Part model, mm, in its own coordinate system. A direction names the side the tool comes from. Give positions to 0.01 mm unless a question says otherwise; leave off trailing zeros. Loops run counter-clockwise (first coordinate to the right, second up) from the corner with the lowest first, then second, coordinate; pieces in that order, holes last. Notation, with made-up numbers: M -20.5,-14.75 L 17.5,-14.75 A20 ccw 17.5,6.25 Z; hole C -14,63 d10. An arc over 180 degrees is marked long. Answer in a Markdown table with one row per item.
from build123d import *

# Parameters (mm, degrees)
CROQUIS1_R              = 3.175
SALIENTE_EXTRUIR1_DEPTH = 150
REDONDEO1_R             = 10
CORTAR_EXTRUIR1_DEPTH   = 13
REDONDEO2_R             = 5
CROQUIS3_W              = 98.791812306
CROQUIS3_H              = 18.145434914
CORTAR_EXTRUIR2_DEPTH   = 13.0000001
CORTAR_EXTRUIR3_DEPTH   = 3.0000001


with BuildPart() as part:
    # Croquis1 → Saliente-Extruir1 (new body)
    with BuildSketch(Plane.XY):
        with BuildLine():
            Line((-2, 19.285827964), (-8.98691391, 23.296314259))
            ThreePointArc((-8.98691391, 23.296314259), (-9.006535925, 33.69237342), (0, 28.5))
            Line((0, 28.5), (0, -28.5))
            ThreePointArc((0, -28.5), (-9.006535925, -33.69237342), (-8.98691391, -23.296314259))
            Line((-8.98691391, -23.296314259), (-2, -19.285827964))
            Line((-2, -19.285827964), (-2, 19.285827964))
        make_face()
        with Locations((-6, 28.5)):
            Circle(CROQUIS1_R, mode=Mode.SUBTRACT)
        with Locations((-6, -28.5)):
            Circle(CROQUIS1_R, mode=Mode.SUBTRACT)
    extrude(amount=-SALIENTE_EXTRUIR1_DEPTH)

    # Redondeo1
    redondeo1_edges = [part.edges().sort_by_distance(p)[0] for p in [
        (-2, -19.285827964, -75),
        (-2, 19.285827964, -75),
    ]]
    fillet(redondeo1_edges, radius=REDONDEO1_R)

    # Croquis2 → Cortar-Extruir1 (cut, through all)
    with BuildSketch(Plane(origin=(0, 0, 0), x_dir=(0, 0, -1), z_dir=(1, 0, 0))):
        Polygon((16, 25), (20, 15.646846929), (20, -15.646846929), (16, -25), (-29.873538988, -25), (-29.873538988, 25), align=None)
    extrude(amount=-CORTAR_EXTRUIR1_DEPTH, mode=Mode.SUBTRACT)

    # Redondeo2
    redondeo2_edges = [part.edges().sort_by_distance(p)[0] for p in [
        (-1.117074127, 15.646846929, -20),
        (-1.117074127, -15.646846929, -20),
        (-5.436698586, -25, -16),
        (-5.436698586, 25, -16),
    ]]
    fillet(redondeo2_edges, radius=REDONDEO2_R)

    # Croquis3 → Cortar-Extruir2 (cut, through all)
    with BuildSketch(Plane(origin=(0, 0, 0), x_dir=(0, 0, -1), z_dir=(1, 0, 0))):
        with Locations((75, 35.875128035)):
            Rectangle(CROQUIS3_W, CROQUIS3_H)
        with Locations((75, -35.875128035)):
            Rectangle(CROQUIS3_W, CROQUIS3_H)
    extrude(amount=-CORTAR_EXTRUIR2_DEPTH, mode=Mode.SUBTRACT)

    # Croquis4 → Cortar-Extruir3 (cut, through all)
    with BuildSketch(Plane.ZY.offset(2)):
        with BuildLine():
            Line((-143.359821197, 3), (-139.627206237, 3))
            ThreePointArc((-139.627206237, 3), (-136.627206237, 0), (-139.627206237, -3))
            Line((-139.627206237, -3), (-143.359821197, -3))
            ThreePointArc((-143.359821197, -3), (-146.359821197, 0), (-143.359821197, 3))
        make_face()
    extrude(amount=-CORTAR_EXTRUIR3_DEPTH, mode=Mode.SUBTRACT)


solid = part.part
(1) Drill centre lines: line 1 along Y through (x, z) = (-5.75, -136.5); line 2 along Z through (x, y) = (-2.5, 27.5); line 3 along Y through (x, z) = (-6, -95) (3 decimals). Where is each one in solid material? Low to high.
Recorded:
| item | result |
|---|---|
| line 1 | y = -34.49 to -31.67, -25.33 to -21.3, 21.3 to 25.33, 31.67 to 34.49 |
| line 2 | z = -150 to -124.4, -25.6 to 0 |
| line 3 | y = -25.325 to -21.496, 21.496 to 25.325 |
(2) Pull direction X, two halves, no side cores. Call faces 6 (the face through (-3.4, 18.6, -84.5)), 7 (the face through (-6.41, -25.35, -73.95)), 8 (the face through (-5, -25, -6)): +X half, -X half, draft (parallel to the pull), parting line (faces both ways), or undercut.
Recorded:
| item | result |
|---|---|
| face 6 | -X half |
| face 7 | undercut |
| face 8 | draft |
(3) Pin check, flat tips, straight feed: pin 1 Ø3 at (x, z) = (-7, -118) entering from +Y; pin 2 Ø0.6 at (x, z) = (-1, -141.5) entering from +Y; pin 3 Ø1.5 at (x, z) = (-9.5, -98) entering from -Y; pin 4 Ø12 at (y, z) = (-12.5, -78) entering from +X. Stop position of each tip, or through.
Recorded:
| item | result |
|---|---|
| pin 1 | stops at y = 26.54 |
| pin 2 | stops at y = 32.23 |
| pin 3 | stops at y = -26.8 |
| pin 4 | stops at x = 0 |
(4) Saw through at B-B (z = -24). Write the cut outline in (x, y) (3 decimals).
Recorded:
| item | result |
|---|---|
| outline | M -8.987,-23.296 A6 ccw long 0,-28.5 L 0,28.5 A6 ccw long -8.987,23.296 L -7.022,22.168 A10 cw -2,13.496 L -2,-13.496 A10 cw -7.022,-22.168 Z; hole C -6,-28.5 d6.35; hole C -6,28.5 d6.35 |
(5) Saw through at C-C (x = -5.25). Give the number of separate pieces and of enclosed holes in the cut face, plus the area to 3 significant figures.
Recorded:
| item | result |
|---|---|
| separate pieces | 6 |
| enclosed holes | 0 |
| area | 1,520 mm^2 |
(6) Saw through at A-A (y = 0). Write the cut outline in (x, z).
Recorded:
| item | result |
|---|---|
| outline | M -2,-150 L 0,-150 L 0,-146.36 L -2,-146.36 Z; M -2,-136.63 L 0,-136.63 L 0,-20 L -2,-20 Z |
(7) Saw through at D-D (z = -104). Write the cut outline in (x, y) (3 decimals), plus the area to 3 significant figures.
Recorded:
| item | result |
|---|---|
| outline | M -11.755,-26.802 L -8.683,-26.802 A3.175 cw -3.317,-26.802 L 0,-26.802 L 0,26.802 L -3.317,26.802 A3.175 cw -8.683,26.802 L -11.755,26.802 A6 ccw -8.987,23.296 L -7.022,22.168 A10 cw -2,13.496 L -2,-13.496 A10 cw -7.022,-22.168 L -8.987,-23.296 A6 ccw Z |
| area | 196 mm^2 |
(8) Which spindle directions (+Z, -Z, +X, -X, +Y, -Y) get a long thin tool onto all of the face, cutting with end or side? Do faces 1 (the face through (-3.31, -18.44, -84.53)), 2 (the face through (-2, 26.802, -74)), 3 (the face through (-1.01, 0.07, -136.63)), 4 (the face through (-1.81, -19.837, -18.208)), 5 (the face through (-2, -26.802, -74)). Say none if no direction does.
Recorded:
| item | result |
|---|---|
| face 1 | +Z, -Z, -X |
| face 2 | +X, -X, +Y |
| face 3 | +X, -X |
| face 4 | +Z, +X, -X |
| face 5 | +X, -X, -Y |
